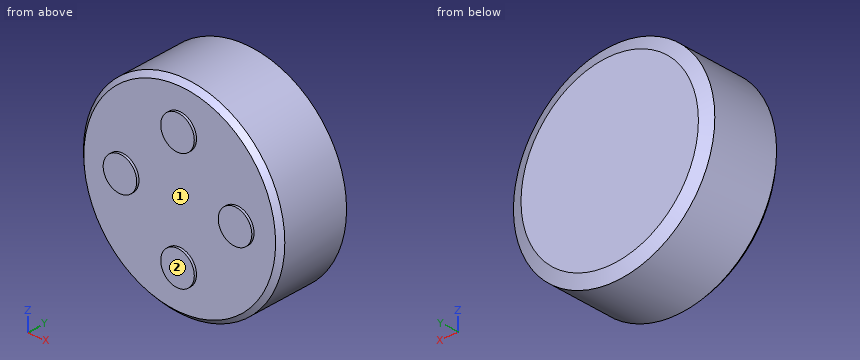
from build123d import *

# Parameters (mm, degrees)
F0_R     = 42
F1_DEPTH = 32
F2_SIZE2 = 5
F2_SIZE  = 2
F3_SIZE  = 2
F4_R     = 7
F5_DEPTH = 1


with BuildPart() as f1:
    # F0 (on Front) → F1 (new body)
    with BuildSketch(Plane.XZ):
        Circle(F0_R)
    extrude(amount=F1_DEPTH)

    # F2
    f2_edges = [f1.edges().sort_by_distance(p)[0] for p in [
        (-42, 0, 0),
    ]]
    chamfer(f2_edges, length=F2_SIZE, length2=F2_SIZE2)

    # F3
    f3_edges = [f1.edges().sort_by_distance(p)[0] for p in [
        (-42, -32, 0),
    ]]
    chamfer(f3_edges, length=F3_SIZE)

    # F4 (on face) → F5 (join)
    with BuildSketch(Plane.XZ.offset(32)):
        with Locations((-24, 0)):
            Circle(F4_R)
        with Locations((24, 0)):
            Circle(F4_R)
        with Locations((0, 24)):
            Circle(F4_R)
        with Locations((0, -24)):
            Circle(F4_R)
    extrude(amount=F5_DEPTH)


solid = f1.part
Input: part model. Units: mm. Frame: model coordinates. Face numbers are marked on the shaded views. A direction names the side the tool comes from. Give positions to 0.01 mm unless a question says otherwise; leave off trailing zeros. Loops run counter-clockwise (first coordinate to the right, second up) from the corner with the lowest first, then second, coordinate; pieces in that order, holes last. Notation, with made-up numbers: (66, -31.75) - (84, -31.75) arc R24 ccw to (84, -5.75) - close; hole circle Ø3 at (-9, 66.5). An arc over 180 degrees is marked (long way). Use CSV: the item, a comma, the result in double quotes. Start each with the question number.
Item 1: Contact query for flat-ended pins moving along their axis: P1, Ø4, axis at y = -16, z = 5, coming from the +X side; P2, Ø12, axis at x = 13, y = -6.5, coming from the -Z side; P3, Ø4, axis at x = -26, y = -25.5, coming from the -Z side. Output: stop coordinate, or through.
Item 2: Reachability of the marked faces 1 and 2 from +Z, -Z, +X, -X, +Y, -Y: full face, straight path, thin tool, end or side. Return the list, or none.
Item 3: Section A-A on y = -18. Return loops of the section in (x, z).
Item 4: Line query: line 1 (X direction, y = -23.5, z = -0.5); line 2 (X direction, y = -30.5, z = 11). Output: solid intervals per line, ascending.
Ans:
1,P1,"stops at x = 41.89"
1,P2,"stops at z = -41.41"
1,P3,"stops at z = -34.47"
2,face 1,"-Y"
2,face 2,"+Z, -Z, +X, -X, -Y"
3,outline,"circle Ø84 at (0, 0)"
4,line 1,"x = -42 to 42"
4,line 2,"x = -40.02 to 40.02"
